Work out the finished part from the listing and answer in its coordinate system (mm). A direction names the side the tool comes from. Round coordinates to 2 decimals unless told otherwise and drop trailing zeros. Write each loop counter-clockwise with the first axis right and the second up, starting at its lowest first coordinate (ties: lowest second). Pieces come first, ordered by that corner, then holes. Notation, with made-up numbers: (-24, 9) -> (6, 9) arc R7 cw to (6, 16) -> close; hole circle Ø3 at (-31, 82.25). An arc over 180 degrees is marked (long way). One line per item, written item: value.
```python
from build123d import *

# Parameters (mm, degrees)
BOSS_EXTRUDE1_DEPTH      = 5
BOSS_EXTRUDE1_DEPTH_BACK = 5
CUT_EXTRUDE1_DEPTH       = 5
BOSS_EXTRUDE2_START      = -14
SKETCH3_W                = 5.881583951
SKETCH3_H                = 10
BOSS_EXTRUDE2_DEPTH      = 8
BOSS_EXTRUDE3_START      = 10
BOSS_EXTRUDE3_DEPTH      = 10
FILLET2_R                = 5
FILLET3_R                = 2
SKETCH5_R                = 2
SKETCH5_W                = 3
SKETCH5_H                = 3
CUT_EXTRUDE2_DEPTH       = 4
FILLET4_R                = 1
SKETCH6_R                = 3.25
CUT_EXTRUDE3_DEPTH       = 5
BOSS_EXTRUDE4_START      = -14
SKETCH7_R                = 2
BOSS_EXTRUDE4_DEPTH      = 3.7
FILLET5_R                = 1.6


with BuildPart() as part:
    # Sketch1 → Boss-Extrude1 (new, two sides: drawn at the far end of the back side and taken through both)
    with BuildSketch(Plane.XY.offset(-BOSS_EXTRUDE1_DEPTH_BACK)):
        Polygon((5, -10), (5, 0), (0, 0), (-5, 0), (-35, 0), (-40, 0), (-40, -14), (-31.982625312, -14), (-31.982625312, -10), (-5, -10), align=None)
        with BuildLine():
            ThreePointArc((-25.78623506, -6.579298906), (-34.5, -5), (-25.78623506, -3.420701094))
            Line((-25.78623506, -3.420701094), (-13.21376494, -3.420701094))
            ThreePointArc((-13.21376494, -3.420701094), (-8.197485897, -0.572136959), (-4.5, -5))
            ThreePointArc((-4.5, -5), (-8.197485897, -9.427863041), (-13.21376494, -6.579298906))
            Line((-13.21376494, -6.579298906), (-25.78623506, -6.579298906))
        make_face(mode=Mode.SUBTRACT)
    extrude(amount=BOSS_EXTRUDE1_DEPTH + BOSS_EXTRUDE1_DEPTH_BACK)

    # Sketch2 → Cut-Extrude1 (cut)
    with BuildSketch(Plane(origin=(0, 0, 0), x_dir=(1, 0, 0), z_dir=(0, 1, 0))):
        with BuildLine():
            Line((-2.520975228, 1.25), (2.520975228, 1.25))
            ThreePointArc((2.520975228, 1.25), (3.770975228, 0), (2.520975228, -1.25))
            Line((2.520975228, -1.25), (-2.520975228, -1.25))
            ThreePointArc((-2.520975228, -1.25), (-3.770975228, 0), (-2.520975228, 1.25))
        make_face()
    extrude(amount=-CUT_EXTRUDE1_DEPTH, mode=Mode.SUBTRACT)

    # Sketch3 → Boss-Extrude2 (add)
    with BuildSketch(Plane(origin=(0, 0, 0), x_dir=(1, 0, 0), z_dir=(0, 1, 0)).offset(BOSS_EXTRUDE2_START)):
        with BuildLine():
            Line((0, 20), (0, 5))
            Line((0, 5), (5.881583951, 5))
            Line((5.881583951, 5), (5.881583951, -5))
            Line((5.881583951, -5), (0, -5))
            Line((0, -5), (0, -20))
            ThreePointArc((0, -20), (14.142135624, -14.142135624), (20, 0))
            ThreePointArc((20, 0), (14.142135624, 14.142135624), (0, 20))
        make_face()
        with Locations((2.940791976, 0)):
            Rectangle(SKETCH3_W, SKETCH3_H)
        with BuildLine():
            Line((0, 5), (-19.364916731, 5))
            ThreePointArc((-19.364916731, 5), (-20, 0), (-19.364916731, -5))
            Line((-19.364916731, -5), (0, -5))
            Line((0, -5), (0, 5))
        make_face()
        with BuildLine():
            Line((-19.364916731, 5), (-40, 5))
            Line((-40, 5), (-40, -5))
            Line((-40, -5), (-19.364916731, -5))
            ThreePointArc((-19.364916731, -5), (-20, 0), (-19.364916731, 5))
        make_face()
    extrude(amount=-BOSS_EXTRUDE2_DEPTH)

    # Sketch4 → Boss-Extrude3 (add)
    with BuildSketch(Plane(origin=(0, -14, 0), x_dir=(1, 0, 0), z_dir=(0, 1, 0)).offset(BOSS_EXTRUDE3_START)):
        with BuildLine():
            ThreePointArc((20, 0), (14.142135624, 14.142135624), (0, 20))
            Line((0, 20), (0, 6))
            Line((0, 6), (6, 6))
            Line((6, 6), (6, -6))
            Line((6, -6), (0, -6))
            Line((0, -6), (0, -20))
            ThreePointArc((0, -20), (14.142135624, -14.142135624), (20, 0))
        make_face()
    extrude(amount=-BOSS_EXTRUDE3_DEPTH)

    # Fillet2
    fillet2_edges = [part.edges().sort_by_distance(p)[0] for p in [
        (-40, -11, -5),
        (-40, -11, 5),
        (6, -9, 6),
        (6, -9, -6),
        (5, -5, 5),
        (5, -5, -5),
    ]]
    fillet(fillet2_edges, radius=FILLET2_R - 0.0001)  # a hair under: the kernel refuses the full size

    # Fillet3
    fillet3_edges = [part.edges().sort_by_distance(p)[0] for p in [
        (-19.5, -3.420701094, 5),
        (-19.5, -3.420701094, -5),
        (-19.5, -6.579298906, 5),
        (-19.5, -6.579298906, -5),
        (-31.982625312, -10, 0),
        (-31.982625312, -14, 0),
        (0, -13, -20),
        (0, -13, 20),
    ]]
    fillet(fillet3_edges, radius=FILLET3_R - 0.0001)  # a hair under: the kernel refuses the full size

    # Sketch5 → Cut-Extrude2 (cut)
    with BuildSketch(Plane.XZ.offset(22)):
        with Locations(Location((0, 0, 0), (0, 0, 270))):
            Circle(SKETCH5_R)
        with BuildLine():
            Line((-35, 3.25), (-12, 3.25))
            ThreePointArc((-12, 3.25), (-8.75, 0), (-12, -3.25))
            Line((-12, -3.25), (-35, -3.25))
            ThreePointArc((-35, -3.25), (-38.25, 0), (-35, 3.25))
        make_face()
        with Locations((-5, 0)):
            Rectangle(SKETCH5_W, SKETCH5_H)
        with Locations((5, 0)):
            Rectangle(SKETCH5_W, SKETCH5_H)
    extrude(amount=-CUT_EXTRUDE2_DEPTH, mode=Mode.SUBTRACT)

    # Fillet4
    fillet4_edges = [part.edges().sort_by_distance(p)[0] for p in [
        (-23.5, -18, 3.25),
        (-8.75, -18, 0),
        (-23.5, -18, -3.25),
        (-38.25, -18, 0),
        (0, -18, -5),
        (0, -18, 5),
        (0, -22, 2),
    ]]
    fillet(fillet4_edges, radius=FILLET4_R)

    # Sketch6 → Cut-Extrude3 (cut)
    with BuildSketch(Plane.XZ.offset(22)):
        with Locations(Location((-35, 0, 0), (0, 0, 270))):
            Circle(SKETCH6_R)
    extrude(amount=-CUT_EXTRUDE3_DEPTH, mode=Mode.SUBTRACT)

    # Sketch7 → Boss-Extrude4 (add)
    with BuildSketch(Plane(origin=(0, 0, 0), x_dir=(1, 0, 0), z_dir=(0, 1, 0)).offset(BOSS_EXTRUDE4_START)):
        with Locations(Location((0, 0, 0), (0, 0, 90))):
            Circle(SKETCH7_R)
    extrude(amount=BOSS_EXTRUDE4_DEPTH)

    # Fillet5
    fillet5_edges = [part.edges().sort_by_distance(p)[0] for p in [
        (0, -14, 2),
        (0, -10.3, 2),
    ]]
    fillet(fillet5_edges, radius=FILLET5_R)


solid = part.part
```
(1) For a pull along Y with two mould halves and no side action, classify faces 4 (the face through (5, -18, 0)), 5 (the face through (0, -13, 12)), 6 (the face through (-20, -3.421, 0)) as pulls with the +Y half, pulls with the -Y half, needs draft (parallel to the pull), parting line crosses it, or undercut.
Reported:
face 4: pulls with the -Y half
face 5: needs draft
face 6: undercut
(2) Find section A-A on x = -23. Give the vertices of the cut face in (y, z), plus the area to 3 significant figures.
Reported:
outline: (-22, -5) -> (-14, -5) -> (-14, 5) -> (-22, 5) -> (-22, 3.25) -> (-19, 3.25) arc R1 cw to (-18, 2.25) -> (-18, -2.25) arc R1 cw to (-19, -3.25) -> (-22, -3.25) -> close; (-10, -5) -> (-8.58, -5) arc R2 ccw to (-6.58, -3) -> (-6.58, 3) arc R2 ccw to (-8.58, 5) -> (-10, 5) -> close; (-3.42, -3) arc R2 ccw to (-1.42, -5) -> (0, -5) -> (0, 5) -> (-1.42, 5) arc R2 ccw to (-3.42, 3) -> close
area: 119 mm2
(3) Find section B-B on y = -2.25. Give the number of separate pieces and of enclosed holes in the cut face, plus the area to 3 significant figures.
Reported:
separate pieces: 3
enclosed holes: 1
area: 264 mm2
(4) Find section C-C on z = -12. Give the vertices of the cut face in (x, y), plus the area to 3 significant figures.
Reported:
outline: (0, -22) -> (16, -22) -> (16, -4) -> (0, -4) -> close
area: 288 mm2
(5) A tool of negligible diameter and unlimited length cuts with its end or side. For faces 1 (the face through (-12, -14, 0)), 2 (the face through (-24, -21, 3.25)), 3 (the face through (-19.39, -2.82, 4.43)), from which of +Z, -Z, +X, -X, +Y, -Y can it reach the whole face along a straight path? Write none if from no direction.
Reported:
face 1: none
face 2: -Y
face 3: +Z
(6) Flat-ended cylindrical pins translate along their axes: pin 1 Ø0.8 at (x, y) = (0.5, -10) entering from +Z; pin 2 Ø2.5 at (x, y) = (-5.5, -19) entering from +Z; pin 3 Ø1.5 at (x, y) = (5.5, -19.5) entering from +Z. Find the tip coordinate at first contact, or state that the pin passes through.
Reported:
pin 1: stops at z = 19.56
pin 2: stops at z = 5
pin 3: stops at z = 19.43
(7) Consider probe 1 along X at (y, z) = (-19, 0); probe 2 along X at (y, z) = (-17.8, 0); probe 3 along Z at (x, y) = (-23, -19.5). Determine where each line is inside the solid, lowest interval first.
Reported:
probe 1: x = -40 to -38.25, -8.75 to -6.5, -3.5 to -2, 2 to 3.5, 6.5 to 20
probe 2: x = -40 to -38.25, -31.75 to 20
probe 3: z = -5 to -3.25, 3.25 to 5
